from build123d import *

# Parameters (mm, degrees)
SKETCH2_R          = 31.049864635
SKETCH2_R_2        = 29.352746911
CUT_EXTRUDE1_DEPTH = 1.5
CUT_EXTRUDE2_DEPTH = 1.5
SKETCH4_R          = 10
CUT_EXTRUDE3_DEPTH = 15


with BuildPart() as part:
    # Sketch1 → Revolve1 (revolve)
    with BuildSketch(Plane.XY, mode=Mode.PRIVATE) as revolve1_sk:
        with BuildLine():
            Line((0, 0), (0, 150))
            Line((0, 150), (30, 150))
            ThreePointArc((30, 150), (40.388997365, 139.611002635), (30, 129.22200527))
            Line((30, 129.22200527), (15, 129.22200527))
            ThreePointArc((15, 129.22200527), (18.060262967, 67.017481004), (10.681483474, 5.176380902))
            Line((10.681483474, 5.176380902), (30, 0))
            Line((30, 0), (0, 0))
        make_face()
    revolve(revolve1_sk.sketch.rotate(Axis((0, 0, 0), (0, 1, 0)), 90), axis=Axis((0, 0, 0), (0, 1, 0)))

    # Sketch2 → Cut-Extrude1 (cut)
    with BuildSketch(Plane(origin=(0, 150, 0), x_dir=(1, 0, 0), z_dir=(0, 1, 0))):
        with Locations(Location((0, 0, 0), (0, 0, 270))):
            Circle(SKETCH2_R)
        with Locations(Location((0, 0, 0), (0, 0, 270))):
            Circle(SKETCH2_R_2, mode=Mode.SUBTRACT)
    extrude(amount=-CUT_EXTRUDE1_DEPTH, mode=Mode.SUBTRACT)

    # Sketch3 → Cut-Extrude2 (cut)
    with BuildSketch(Plane(origin=(0, 150, 0), x_dir=(1, 0, 0), z_dir=(0, 1, 0))):
        with BuildLine():
            Line((-1.37380559, 11.490731507), (0.200524373, 11.490731507))
            Line((0.200524373, 11.490731507), (9.720590268, -5.252730688))
            add(Edge.make_bspline(
                [(9.720590268, -5.252730688), (9.775425809, -5.336848559), (9.884824755, -5.504666839), (10.109686394, -5.712624674), (10.364541879, -5.897673839), (10.667511649, -6.039567124), (11.004675554, -6.156309685), (11.38520549, -6.229119021), (11.802008113, -6.284806014), (12.094830032, -6.288182504), (12.24692682, -6.289936311)],
                knots=[0, 0, 0, 0, 0.840177971, 1.676186298, 2.553734707, 3.476611938, 4.473478221, 5.543186981, 6.723888672, 8, 8, 8, 8], degree=3))
            Line((12.24692682, -6.289936311), (13.135960211, -6.289936311))
            Line((13.135960211, -6.289936311), (13.135960211, -7.238238595))
            Line((13.135960211, -7.238238595), (1.756332807, -7.238238595))
            Line((1.756332807, -7.238238595), (1.756332807, -6.289936311))
            Line((1.756332807, -6.289936311), (2.663887727, -6.289936311))
            add(Edge.make_bspline(
                [(2.663887727, -6.289936311), (2.80588403, -6.289116844), (3.080045555, -6.287534645), (3.475468257, -6.278554582), (3.838258818, -6.253484746), (4.168672223, -6.231533819), (4.464628818, -6.191836085), (4.72989755, -6.153782934), (4.962737436, -6.103045308), (5.105277775, -6.058706001), (5.171702751, -6.038043517)],
                knots=[0, 0, 0, 0, 1.347381447, 2.601477244, 3.751787047, 4.797723897, 5.742291361, 6.584045584, 7.340153537, 8, 8, 8, 8], degree=3))
            add(Edge.make_bspline(
                [(5.171702751, -6.038043517), (5.246729637, -6.008546001), (5.384240305, -5.954482408), (5.546196056, -5.82449007), (5.656795371, -5.670049367), (5.666823825, -5.551932666), (5.671784033, -5.493510565)],
                knots=[0, 0, 0, 0, 1.216663799, 2.229923951, 3.124496705, 4, 4, 4, 4], degree=3))
            add(Edge.make_bspline(
                [(5.671784033, -5.493510565), (5.664990337, -5.418196965), (5.650521617, -5.25779954), (5.577280328, -5.114104756), (5.538429024, -5.037880952)],
                knots=[0, 0, 0, 0, 0.939087396, 2, 2, 2, 2], degree=3))
            Line((5.538429024, -5.037880952), (3.278802489, -1.074273751))
            Line((3.278802489, -1.074273751), (-7.474797235, -1.074273751))
            Line((-7.474797235, -1.074273751), (-8.852798991, -3.34871751))
            add(Edge.make_bspline(
                [(-8.852798991, -3.34871751), (-8.928421945, -3.490696961), (-9.068680664, -3.754027804), (-9.224116161, -4.138619247), (-9.332642883, -4.475115772), (-9.346569932, -4.68905318), (-9.352880274, -4.785988158)],
                knots=[0, 0, 0, 0, 1.256117806, 2.329735437, 3.2432036, 4, 4, 4, 4], degree=3))
            add(Edge.make_bspline(
                [(-9.352880274, -4.785988158), (-9.343177226, -4.888324501), (-9.323371536, -5.097211653), (-9.141155652, -5.38324454), (-8.868849037, -5.641461835), (-8.567657199, -5.824455709), (-8.282154901, -5.959469659), (-8.032782233, -6.045389303), (-7.761909609, -6.126127912), (-7.464752755, -6.181705917), (-7.144821029, -6.230173712), (-6.801442809, -6.26855562), (-6.43280877, -6.284674672), (-6.179532542, -6.288143581), (-6.048639504, -6.289936311)],
                knots=[0, 0, 0, 0, 0.925715885, 1.889555053, 3.00451202, 4.335528446, 5.081180176, 5.882656101, 6.738094346, 7.656865631, 8.636367395, 9.689735017, 10.806056124, 12, 12, 12, 12], degree=3))
            Line((-6.048639504, -6.289936311), (-5.118858749, -6.289936311))
            Line((-5.118858749, -6.289936311), (-5.118858749, -7.238238595))
            Line((-5.118858749, -7.238238595), (-15.076032728, -7.238238595))
            Line((-15.076032728, -7.238238595), (-15.076032728, -6.289936311))
            add(Edge.make_bspline(
                [(-15.076032728, -6.289936311), (-14.820152301, -6.284911472), (-14.335067052, -6.275385635), (-13.649411461, -6.18740497), (-13.047349106, -6.042660349), (-12.51508477, -5.832556662), (-12.035352921, -5.529178123), (-11.593750012, -5.122125622), (-11.164977743, -4.615349339), (-10.919691242, -4.222803331), (-10.790150922, -4.015492553)],
                knots=[0, 0, 0, 0, 1.192324888, 2.260349586, 3.215193263, 4.072390854, 4.915560629, 5.844785241, 6.861791383, 8, 8, 8, 8], degree=3))
            Line((-10.790150922, -4.015492553), (-1.37380559, 11.490731507))
        make_face()
        Polygon((-1.918338542, 8.075361564), (-6.900629837, -0.125971467), (2.741678149, -0.125971467), align=None, mode=Mode.SUBTRACT)
    extrude(amount=-CUT_EXTRUDE2_DEPTH, mode=Mode.SUBTRACT)

    # Sketch4 → Cut-Extrude3 (cut)
    with BuildSketch(Plane(origin=(0, 0, 0), x_dir=(-1, 0, 0), z_dir=(0, -1, 0))):
        with Locations(Location((0, 0, 0), (0, 0, 90))):
            Circle(SKETCH4_R)
    extrude(amount=-CUT_EXTRUDE3_DEPTH, mode=Mode.SUBTRACT)


solid = part.part
Here's how the part is built. I have some questions about the finished solid (model axes, mm). A direction names the side the tool comes from. Give positions to 0.01 mm unless a question says otherwise; leave off trailing zeros. Use a Markdown table: item, result. Add a question column.
Item 1: If we mould it in two halves opening along X, with no side actions, what happens to faces 5 (the face through (0, 0, -13)), 6 (the face through (-3.571, 4.853, -11.341)), 7 (the face through (4.89, 149.26, -3.24))? For each: pulls with the +X half, pulls with the -X half, needs draft (parallel to the pull), parting line crosses it, or undercut.
Item 2: Will these pins go through, and if not, where does the flat tip stop? pin 1 (2 mm diameter, centred on x = -20.5, z = 11, fed in from -Y); pin 2 (0.8 mm diameter, centred on x = -0.5, y = 149, fed in from +Z); pin 3 (1 mm diameter, centred on x = -4, y = 19, fed in from +Z) (3 decimals); pin 4 (1 mm diameter, centred on y = 149.5, z = 6.5, fed in from +X).
Item 3: I need wall thicknesses on line 1 (X direction, y = 149, z = 0); line 2 (Y direction, x = 13, z = -19.5); line 3 (Y direction, x = 23, z = 15). Which ranges of each line are inside material? Lowest first, please.
Item 4: For faces 1 (the face through (19, 148.5, 23)), 2 (the face through (-9.76, 7.4, 2.17)), 3 (the face through (0, 150, 6)), 4 (the face through (-14, 129.222, -6)), which set-ups out of +Z, -Z, +X, -X, +Y, -Y let a thin tool reach every point of the face, with its end or its side?
Data:
| question | item | result |
|---|---|---|
| 1 | face 5 | needs draft |
| 1 | face 6 | parting line crosses it |
| 1 | face 7 | undercut |
| 2 | pin 1 | stops at y = 0 |
| 2 | pin 2 | stops at z = 35.21 |
| 2 | pin 3 | stops at z = 12.805 |
| 2 | pin 4 | stops at x = 33.83 |
| 3 | line 1 | x = -34.45 to -31.05, -29.35 to -8.35, -6.82 to 2.67, 6.73 to 29.35, 31.05 to 34.45 |
| 3 | line 2 | y = 0 to 1.76, 129.22 to 150 |
| 3 | line 3 | y = 0 to 0.68, 129.22 to 150 |
| 4 | face 1 | +Y |
| 4 | face 2 | -Y |
| 4 | face 3 | +Z, -Z, +X, -X, +Y |
| 4 | face 4 | none |
